Geometry check sheet. Reference: the model listing, model coordinates, mm. A direction names the side the tool comes from. Give positions to 0.01 mm unless a question says otherwise; leave off trailing zeros. Write each loop counter-clockwise with the first axis right and the second up, starting at its lowest first coordinate (ties: lowest second). Pieces come first, ordered by that corner, then holes. Notation, with made-up numbers: (62, 43) - (101, 43) arc R23 cw to (101, 76) - close; hole circle Ø3 at (11, -9). An arc over 180 degrees is marked (long way). One line per question, with ' | ' between items. Start each with the question number.
Q1. Section check A-A on x = -17. Record the boundary of the cut face in (y, z), and give its area (3 significant figures).
Q2. Thickness scan on L1, parallel to Y at x = -7, z = 1.75; L2, parallel to Y at x = 28.5, z = 8.25; L3, parallel to Y at x = 27, z = 8.25. Record the ranges inside material, lowest first. Write a range as [from, to].
Q3. Section check B-B on z = 1.5. Record the boundary of the cut face in (x, y).
Q4. Release check for a two-part mould opening along Z. For faces 6 (the face through (30.015, 0.857, 7.34)), 7 (the face through (27, 17, 11.5)), 8 (the face through (-11.19, 24.87, 1.48)) record: +Z half, -Z half, draft (parallel to the pull), parting line (faces both ways), or undercut.
Q5. Set-up check for faces 1 (the face through (13, 23.758, 1)), 2 (the face through (28, -5.467, 8)), 3 (the face through (27.3, 15, 7.7)), 4 (the face through (-33, 21.57, 1)), 5 (the face through (-33.096, 0, 1)): record each of +Z, -Z, +X, -X, +Y, -Y from which the full face is reachable in a straight line by a thin tool's end or side.
Q6. Gauge pin test, flat ends, axial feed: P1, Ø3, axis at y = -0.5, z = 6, coming from the +X side; P2, Ø1.8, axis at x = 29.5, z = 9.5, coming from the -Y side; P3, Ø0.9, axis at x = 4.5, z = 1.5, coming from the +Y side. Record the tip position at first contact, or that the pin passes through.
Q7. Section check C-C on x = 14. Record the boundary of the cut face in (y, z), and give its area (3 significant figures).
```python
from build123d import *

# Parameters (mm, degrees)
SKETCH_2_R          = 2.5
SKETCH_2_R_2        = 4
EXTRUDE_1_DEPTH     = 3
SKETCH_2_3_R        = 4
SKETCH_2_3_R_2      = 2
EXTRUDE_2_DEPTH     = 11.5
SKETCH_6_R          = 2
EXTRUDE_3_DEPTH     = 2.3
FILLET_1_R          = 2
SKETCH_7_R          = 2.5
SKETCH_7_R_2        = 2
CUT_EXTRUDE_2_DEPTH = 2
FILLET_2_R          = 1


with BuildPart() as part:
    # Sketch 2 → Extrude 1 (new body)
    with BuildSketch(Plane.XY):
        Polygon((-41.138288377, 15.425110404), (-41.138288377, 21.570131373), (-25.053133429, 21.570131373), (-20.677655191, 25.94560961), (-13.728698976, 25.94560961), (-8.574109119, 23.757870491), (35.231937864, 23.757870491), (41.138288377, 21.251065018), (41.138288377, -25.94560961), (-41.138288377, -25.94560961), (-41.138288377, -12.020899542), (-33.095710903, -12.020899542), (-33.095710903, 11.403821667), (-37.11699964, 11.403821667), align=None)
        with Locations((10.421946091, 8.532959579)):
            Circle(SKETCH_2_R, mode=Mode.SUBTRACT)
        with Locations((-7.306059133, -18.107570273)):
            Circle(SKETCH_2_R, mode=Mode.SUBTRACT)
        with Locations((25.421946091, 18.532959579)):
            Circle(SKETCH_2_R_2, mode=Mode.SUBTRACT)
        with Locations((-28.314407571, 7.976729123)):
            Circle(SKETCH_2_R_2, mode=Mode.SUBTRACT)
        with Locations((-17, 20.7)):
            Circle(SKETCH_2_R, mode=Mode.SUBTRACT)
        with BuildLine():
            Line((25.543402205, -5.467040421), (31.421946091, -5.467040421))
            ThreePointArc((31.421946091, -5.467040421), (32.129052872, -5.174147202), (32.421946091, -4.467040421))
            Line((32.421946091, -4.467040421), (32.421946091, 1.411503465))
            ThreePointArc((32.421946091, 1.411503465), (32.076213917, 2.167766389), (31.278078869, 2.401100465))
            ThreePointArc((31.278078869, 2.401100465), (26.799843583, 0.155062087), (24.553805205, -4.323173199))
            ThreePointArc((24.553805205, -4.323173199), (24.78713928, -5.121308248), (25.543402205, -5.467040421))
        make_face(mode=Mode.SUBTRACT)
    extrude(amount=EXTRUDE_1_DEPTH)

    # Sketch 2_3 → Extrude 2 (add)
    # profile 1 of 3: a face of its own
    with BuildSketch(Plane.XY):
        with Locations((-28.314407571, 7.976729123)):
            Circle(SKETCH_2_3_R)
        with Locations((-28.314407571, 7.976729123)):
            Circle(SKETCH_2_3_R_2, mode=Mode.SUBTRACT)
    # profile 2 of 3: a face of its own
    with BuildSketch(Plane.XY):
        with Locations((25.421946091, 18.532959579)):
            Circle(SKETCH_2_3_R)
        with Locations((25.421946091, 18.532959579)):
            Circle(SKETCH_2_3_R_2, mode=Mode.SUBTRACT)
    # profile 3 of 3: a face of its own
    with BuildSketch(Plane.XY):
        with BuildLine():
            Line((25.543402205, -5.467040421), (31.421946091, -5.467040421))
            ThreePointArc((31.421946091, -5.467040421), (32.129052872, -5.174147202), (32.421946091, -4.467040421))
            Line((32.421946091, -4.467040421), (32.421946091, 1.411503465))
            ThreePointArc((32.421946091, 1.411503465), (32.076213917, 2.167766389), (31.278078869, 2.401100465))
            ThreePointArc((31.278078869, 2.401100465), (26.799843583, 0.155062087), (24.553805205, -4.323173199))
            ThreePointArc((24.553805205, -4.323173199), (24.78713928, -5.121308248), (25.543402205, -5.467040421))
        make_face()
        with Locations((29.464448227, -2.509542558)):
            Circle(SKETCH_2_3_R_2, mode=Mode.SUBTRACT)
    extrude(amount=EXTRUDE_2_DEPTH)

    # Sketch 6 → Extrude 3 (add, symmetric)
    with BuildSketch(Plane(origin=(1.480786333, -5.526369829, 0), x_dir=(0, 0, 1), z_dir=(-0.25881904510252574, 0.9659258262890671, 0))):
        with Locations(Location((7.25, 26.715994864, 0), (0, 0, 90))):
            Circle(SKETCH_6_R)
    extrude(amount=EXTRUDE_3_DEPTH, both=True)

    # Fillet 1
    fillet_1_edges = [part.edges().sort_by_distance(p)[0] for p in [
        (24.75932029, 3.092229761, 7.25),
    ]]
    fillet(fillet_1_edges, radius=FILLET_1_R)

    # Sketch 7 → Cut-Extrude 2 (cut)
    with BuildSketch(Plane(origin=(1.480786333, -5.526369829, 0), x_dir=(0, 0, 1), z_dir=(-0.25881904510252574, 0.9659258262890671, 0))):
        with Locations((7.25, 26.715994864)):
            Circle(SKETCH_7_R)
        with Locations(Location((7.25, 26.715994864, 0), (0, 0, 270))):
            Circle(SKETCH_7_R_2, mode=Mode.SUBTRACT)
    extrude(amount=-CUT_EXTRUDE_2_DEPTH, mode=Mode.SUBTRACT)

    # Fillet 2
    fillet_2_edges = [part.edges().sort_by_distance(p)[0] for p in [
        (32.421946091, -1.527768478, 3),
        (32.129052872, -5.174147202, 3),
        (21.421946091, 18.532959579, 3),
        (-32.314407571, 7.976729123, 3),
        (28.482674148, -5.467040421, 3),
        (24.78713928, -5.121308248, 3),
        (26.799843583, 0.155062087, 3),
        (32.076213917, 2.167766389, 3),
    ]]
    fillet(fillet_2_edges, radius=FILLET_2_R)


solid = part.part
```
Working result:
1) outline: (-25.95, 0) - (18.2, 0) - (18.2, 3) - (-25.95, 3) - close; (23.2, 0) - (25.95, 0) - (25.95, 3) - (23.2, 3) - close | area: 141 mm2
2) L1: y = [-25.95, -20.59], [-15.63, 23.76] | L2: y = [-5.47, -4.26], [-0.76, 2.83], [15.98, 21.09] | L3: y = [-5.47, 3.4], [14.86, 17.3], [19.76, 22.21]
3) outline: (-41.14, -25.95) - (41.14, -25.95) - (41.14, 21.25) - (35.23, 23.76) - (-8.57, 23.76) - (-13.73, 25.95) - (-20.68, 25.95) - (-25.05, 21.57) - (-41.14, 21.57) - (-41.14, 15.43) - (-37.12, 11.4) - (-33.1, 11.4) - (-33.1, -12.02) - (-41.14, -12.02) - close; hole circle Ø4 at (-28.31, 7.98); hole circle Ø5 at (-17, 20.7); hole circle Ø5 at (-7.31, -18.11); hole circle Ø5 at (10.42, 8.53); hole circle Ø4 at (25.42, 18.53); hole circle Ø4 at (29.46, -2.51)
4) face 6: undercut | face 7: +Z half | face 8: draft
5) face 1: +Z, -Z, +X, +Y | face 2: +Z, +X, -X, -Y | face 3: +Z | face 4: +Z, -Z, -X, +Y | face 5: +Z, -Z, -X
6) P1: stops at x = 32.42 | P2: stops at y = -5.47 | P3: stops at y = 23.76
7) outline: (-25.95, 0) - (23.76, 0) - (23.76, 3) - (-25.95, 3) - close | area: 149 mm2
